```python
from build123d import *

# Parameters (mm, degrees)
F0_R     = 1.6
F1_DEPTH = 3


with BuildPart() as f1:
    # F0 (on Top) → F1 (new body)
    with BuildSketch(Plane.XY):
        with BuildLine():
            Line((-19.4697175733, -4.5393385149), (-19.4718945337, -4.5642212863))
            Line((-19.4718945337, -4.5642212863), (-28.1188425534, -103.3992894107))
            Line((-28.1188425534, -103.3992894107), (-9.1911432897, -105.0552485229))
            Line((-9.1911432897, -105.0552485229), (-0.4755690149, -5.4357787137))
            Line((-0.4755690149, -5.4357787137), (-0.0637739547, -0.7289396381))
            ThreePointArc((-0.0637739547, -0.7289396381), (-1.1824461608, 1.8784665345), (-3.9736495146, 2.3875620971))
            Line((-3.9736495146, 2.3875620971), (-17.4024249446, -1.9457712363))
            ThreePointArc((-17.4024249446, -1.9457712363), (-18.8270724233, -2.930893855), (-19.4697175733, -4.5393385149))
        make_face()
        with Locations((-14.8408756973, -9)):
            Circle(F0_R, mode=Mode.SUBTRACT)
        with Locations((-5.5440311689, -6)):
            Circle(F0_R, mode=Mode.SUBTRACT)
    extrude(amount=F1_DEPTH)


solid = f1.part
```
Input: part model. Units: mm. Frame: model coordinates. Round coordinates to 2 decimals unless told otherwise and drop trailing zeros. Loops run counter-clockwise (first coordinate to the right, second up) from the corner with the lowest first, then second, coordinate; pieces in that order, holes last. Notation, with made-up numbers: (-11.75, -13) -> (10.25, -13) arc R24 ccw to (10.25, 26) -> close; hole circle Ø3 at (-7.5, 88). An arc over 180 degrees is marked (long way). Write each question's results on one line, items separated by ' | '.
1. Ray query, line 1 (Y direction, x = -16, z = 1.95); line 2 (X direction, y = -8, z = 2.55); line 3 (Y direction, x = -15, z = 2.85). Return the intervals inside material, ascending. Write a range as from..to.
Geometry results:
line 1: -104.46..-10.1, -7.9..-1.49 | line 2: -19.77..-16.09, -13.59..-0.7 | line 3: -104.55..-10.59, -7.41..-1.17
2. First-contact query: P1, Ø1.5, axis at y = -19.5, z = 2, coming from the -X side; P2, Ø1.5, axis at y = -58, z = 2.5, coming from the +X side; P3, Ø1.5, axis at y = -71, z = 2, coming from the +X side. Flat tips, straight axial feed; report the tip coordinate or a pass-through.
Geometry results:
P1: x = -20.84 | P2: x = -5.01 | P3: x = -6.15
3. Section D-D (x = -8.25). Return loops of the section in (y, z), and give its area (3 significant figures).
Geometry results:
outline: (-94.3, 0) -> (1.01, 0) -> (1.01, 3) -> (-94.3, 3) -> close | area: 286 mm2
4. Section A-A (z = 0.9). Return loops of the section in (x, y).
Geometry results:
outline: (-28.12, -103.4) -> (-9.19, -105.06) -> (-0.06, -0.73) arc R3 ccw to (-3.97, 2.39) -> (-17.4, -1.95) arc R3 ccw to (-19.47, -4.54) -> close; hole circle Ø3.2 at (-14.84, -9); hole circle Ø3.2 at (-5.54, -6)
5. Section C-C (y = -57.5). Return loops of the section in (x, z).
Geometry results:
outline: (-24.1, 0) -> (-5.03, 0) -> (-5.03, 3) -> (-24.1, 3) -> close
6. Mould query, pull axis X, two halves, no side actions, for faces 1 (the face through (-5.891, -7.562, 1.479)), 2 (the face through (-13.36, -9.61, 1.48)), 3 (the face through (-14, -51, 0)), 4 (the face through (-18.787, -104.216, 1.479)). Classes: +X half, -X half, draft (parallel to the pull), parting line (faces both ways), or undercut.
Geometry results:
face 1: undercut | face 2: undercut | face 3: draft | face 4: -X half
7. Section B-B (y = -9). Return loops of the section in (x, z), and give its area (3 significant figures).
Geometry results:
outline: (-19.86, 0) -> (-16.44, 0) -> (-16.44, 3) -> (-19.86, 3) -> close; (-13.24, 0) -> (-0.79, 0) -> (-0.79, 3) -> (-13.24, 3) -> close | area: 47.6 mm2
